The listing builds one solid part. Answer for the finished solid, in the listing's coordinates (mm). A direction names the side the tool comes from. Round coordinates to 2 decimals unless told otherwise and drop trailing zeros. Write each loop counter-clockwise with the first axis right and the second up, starting at its lowest first coordinate (ties: lowest second). Pieces come first, ordered by that corner, then holes. Notation, with made-up numbers: (60.5, 50.5) - (70.5, 50.5) arc R22 cw to (70.5, 66.5) - close; hole circle Ø2 at (-30.75, 20.5). An arc over 180 degrees is marked (long way). Answer in a Markdown table with one row per item.
from build123d import *

# Parameters (mm, degrees)
F1_DEPTH = 38.1
F2_R     = 9.525
F3_R     = 3.175
F4_R     = 9.525
F5_R     = 8.7376
F6_DEPTH = 25.4
F8_DEPTH = 25.4


with BuildPart() as f1:
    # F0 (on Front) → F1 (new body, symmetric)
    with BuildSketch(Plane.XZ):
        Polygon((-193.675, 127), (-203.2, 127), (-203.2, 0), (203.2, 0), (203.2, 9.525), (-193.675, 9.525), align=None)
    extrude(amount=F1_DEPTH, both=True)

    # F2
    f2_edges = [f1.edges().sort_by_distance(p)[0] for p in [
        (-198.4375, -38.1, 127),
        (-198.4375, 38.1, 127),
        (203.2, -38.1, 4.7625),
        (203.2, 38.1, 4.7625),
    ]]
    fillet(f2_edges, radius=F2_R)

    # F3
    f3_edges = [f1.edges().sort_by_distance(p)[0] for p in [
        (-193.675, 0, 9.525),
    ]]
    fillet(f3_edges, radius=F3_R)

    # F4
    f4_edges = [f1.edges().sort_by_distance(p)[0] for p in [
        (-203.2, 0, 0),
    ]]
    fillet(f4_edges, radius=F4_R)

    # F5 (on face) → F6 (cut)
    with BuildSketch(Plane(origin=(-203.2, 0, 0), x_dir=(0, -1, 0), z_dir=(-1, 0, 0))):
        with Locations((20.6248, 101.6)):
            Circle(F5_R)
        with Locations((-20.6248, 31.75)):
            Circle(F5_R)
        with Locations((20.6248, 31.75)):
            Circle(F5_R)
        with Locations((-20.6248, 101.6)):
            Circle(F5_R)
    extrude(amount=-F6_DEPTH, mode=Mode.SUBTRACT)

    # F7 (on face) → F8 (cut)
    with BuildSketch(Plane.XY.offset(9.525)):
        with BuildLine():
            ThreePointArc((-88.9, 8.763), (-97.663, 0), (-88.9, -8.763))
            Line((-88.9, -8.763), (88.9, -8.763))
            ThreePointArc((88.9, -8.763), (97.663, 0), (88.9, 8.763))
            Line((88.9, 8.763), (-88.9, 8.763))
        make_face()
    extrude(amount=-F8_DEPTH, mode=Mode.SUBTRACT)


solid = f1.part
(1) For faces 4 (the cylindrical face through (-198.5, -24.66, 24)), 5 (the flat face through (-193.675, -1, 69)), 6 (the flat face through (1, 8.763, 5)), determine the directions among +Z, -Z, +X, -X, +Y, -Y from which every point of the face is accessible in a straight line to the end or side of a thin tool.
Checked values:
| item | result |
|---|---|
| face 4 | +X, -X |
| face 5 | +Z, +X, +Y, -Y |
| face 6 | +Z, -Z |
(2) A flat-ended cylindrical pin translates along its axis: pin 1 (15.5 mm diameter, centred on y = -20.62, z = 101.6, fed in from -X). Find the tip coordinate at first contact, or state that the pin passes through.
Checked values:
| item | result |
|---|---|
| pin 1 | passes through |
(3) Find the intervals of material crossed by line 1 (Y direction, x = -200, z = 31); line 2 (Z direction, x = 81, y = -24) (3 decimals); line 3 (X direction, y = -26, z = 74.5) (3 decimals), in increasing order.
Checked values:
| item | result |
|---|---|
| line 1 | y = -38.1 to -29.33, -11.92 to 11.92, 29.33 to 38.1 |
| line 2 | z = 0 to 9.525 |
| line 3 | x = -203.2 to -193.675 |
(4) Section C-C (y = -20.5) is taken. Give the vertices of the cut face in (x, z) (3 decimals).
Checked values:
| item | result |
|---|---|
| outline | (-203.2, 9.525) arc R9.525 ccw to (-193.675, 0) - (203.2, 0) - (203.2, 9.525) - (-190.5, 9.525) arc R3.175 cw to (-193.675, 12.7) - (-193.675, 23.013) - (-203.2, 23.013) - close; (-203.2, 40.487) - (-193.675, 40.487) - (-193.675, 92.863) - (-203.2, 92.863) - close; (-203.2, 110.337) - (-193.675, 110.337) - (-193.675, 127) - (-203.2, 127) - close |
(5) Section B-B (x = 81) is taken. Give the vertices of the cut face in (y, z) (3 decimals), and give its area (3 significant figures).
Checked values:
| item | result |
|---|---|
| outline | (-38.1, 0) - (-8.763, 0) - (-8.763, 9.525) - (-38.1, 9.525) - close; (8.763, 0) - (38.1, 0) - (38.1, 9.525) - (8.763, 9.525) - close |
| area | 559 mm2 |
(6) Section D-D (z = 52) is taken. Give the vertices of the cut face in (x, y) (3 decimals), and give its area (3 significant figures).
Checked values:
| item | result |
|---|---|
| outline | (-203.2, -38.1) - (-193.675, -38.1) - (-193.675, 38.1) - (-203.2, 38.1) - close |
| area | 726 mm2 |
(7) Section A-A (z = 31.75) is taken. Give the vertices of the cut face in (x, y) (3 decimals), and give its area (3 significant figures).
Checked values:
| item | result |
|---|---|
| outline | (-203.2, -38.1) - (-193.675, -38.1) - (-193.675, -29.362) - (-203.2, -29.362) - close; (-203.2, -11.887) - (-193.675, -11.887) - (-193.675, 11.887) - (-203.2, 11.887) - close; (-203.2, 29.362) - (-193.675, 29.362) - (-193.675, 38.1) - (-203.2, 38.1) - close |
| area | 393 mm2 |
(8) For a pull along Y with two mould halves and no side action, classify faces 1 (the flat face through (-64, 38.1, 7)), 2 (the cylindrical face through (-198.5, -28.96, 104.22)), 3 (the flat face through (2, -9, 0)) as pulls with the +Y half, pulls with the -Y half, needs draft (parallel to the pull), parting line crosses it, or undercut.
Checked values:
| item | result |
|---|---|
| face 1 | pulls with the +Y half |
| face 2 | undercut |
| face 3 | needs draft |
